Source: CAD feature listing. Evaluate the final solid. Frame: model axes, mm. A direction names the side the tool comes from. Round coordinates to 2 decimals unless told otherwise and drop trailing zeros. Loops run counter-clockwise (first coordinate to the right, second up) from the corner with the lowest first, then second, coordinate; pieces in that order, holes last. Notation, with made-up numbers: M -30.75,44 L -6.75,44 A8 ccw -6.75,58 Z; hole C 65,36.5 d3. An arc over 180 degrees is marked long. One line per item, written item: value.
from build123d import *

# Parameters (mm, degrees)
SKETCH1_R                  = 109.714317711
SKETCH1_R_2                = 85.130943159
BOSS_EXTRUDE1_DEPTH        = 50
BOSS_EXTRUDE2_REACH        = 241.217
BOSS_EXTRUDE2_START_RADIUS = 109.714317711
BOSS_EXTRUDE2_END_RADIUS   = 109.714317711
SKETCH2_W                  = 26
SKETCH2_H                  = 26
SKETCH2_W_2                = 20
SKETCH2_H_2                = 20


with BuildPart() as part:
    # Sketch1 → Boss-Extrude1 (new body)
    with BuildSketch(Plane.XY):
        Circle(SKETCH1_R)
        Circle(SKETCH1_R_2, mode=Mode.SUBTRACT)
    extrude(amount=BOSS_EXTRUDE1_DEPTH)

    # Boss-Extrude2: from a cylinder face, 241.217 long prism both ways, kept between that surface and its translate by the depth
    boss_extrude2_start = Plane(origin=(0, 0, 25), z_dir=(0, 0, -1)) * Cylinder(BOSS_EXTRUDE2_START_RADIUS, 702.862635421, mode=Mode.PRIVATE)
    boss_extrude2_end = Plane(origin=(76.2, 0, 25), z_dir=(0, 0, -1)) * Cylinder(BOSS_EXTRUDE2_END_RADIUS, 702.862635421, mode=Mode.PRIVATE)
    # Sketch2 → Boss-Extrude2 (add, from a surface)
    with BuildSketch(Plane(origin=(0, 0, 0), x_dir=(0, 0, -1), z_dir=(1, 0, 0)), mode=Mode.PRIVATE) as boss_extrude2_sk1:
        with Locations((-25, 0)):
            Rectangle(SKETCH2_W, SKETCH2_H)
        with Locations((-25, 0)):
            Rectangle(SKETCH2_W_2, SKETCH2_H_2, mode=Mode.SUBTRACT)
    boss_extrude2_tool1 = extrude(boss_extrude2_sk1.sketch, amount=BOSS_EXTRUDE2_REACH, both=True, mode=Mode.PRIVATE)
    add(((boss_extrude2_tool1 - boss_extrude2_start) & boss_extrude2_end).solids().sort_by_distance((147.199526, 12.632304, 25))[0])


solid = part.part
1. Section query D-D (x = 0). Return the cut outline in (y, z), and give its area (3 significant figures).
Report:
outline: M -109.71,0 L -85.13,0 L -85.13,50 L -109.71,50 Z; M 85.13,0 L 109.71,0 L 109.71,50 L 85.13,50 Z
area: 2,460 mm2
2. Section query A-A (z = 29). Return the cut outline in (x, y).
Report:
outline: M 108.94,-13 L 185.14,-13 A109.71 ccw 185.46,-10 L 109.26,-10 A109.71 ccw 109.26,10 L 185.46,10 A109.71 ccw 185.14,13 L 108.94,13 A109.71 ccw long Z; hole C 0,0 d170.26
3. Ray query, line 1 (Z direction, x = 173, y = 2); line 2 (Y direction, x = 0, z = 33); line 3 (Y direction, x = 139.5, z = 21.5). Return the intervals inside material, ascending. Write a range as [from, to].
Report:
line 1: z = [12, 15], [35, 38]
line 2: y = [-109.71, -85.13], [85.13, 109.71]
line 3: y = [-13, -10], [10, 13]
4. Section query B-B (x = 163). Return the cut outline in (y, z).
Report:
outline: M -13,12 L 13,12 L 13,38 L -13,38 Z; hole M -10,15 L 10,15 L 10,35 L -10,35 Z
5. Reachability of faces 1 (the face through (148, 0, 15)), 2 (the face through (148, 0, 12)), 3 (the face through (148, 13, 25)) from +Z, -Z, +X, -X, +Y, -Y: full face, straight path, thin tool, end or side. Return the list, or none.
Report:
face 1: +X
face 2: -Z, +X, +Y, -Y
face 3: +Z, -Z, +X, +Y
6. Section query C-C (y = 0). Return the cut outline in (x, z), and give its area (3 significant figures).
Report:
outline: M -109.71,0 L -85.13,0 L -85.13,50 L -109.71,50 Z; M 85.13,0 L 109.71,0 L 109.71,12 L 185.91,12 L 185.91,15 L 109.71,15 L 109.71,35 L 185.91,35 L 185.91,38 L 109.71,38 L 109.71,50 L 85.13,50 Z
area: 2,920 mm2
7. Pin query (flat end, axial travel): pin 1 (1 mm diameter, centred on y = 26, z = 13.5, fed in from -X); pin 2 (10 mm diameter, centred on x = 128.5, z = 27, fed in from -Y); pin 3 (22 mm diameter, centred on x = 152.5, z = 23.5, fed in from +Y). Return the tip coordinate at first contact, or that it passes through.
Report:
pin 1: stops at x = -106.71
pin 2: stops at y = -13
pin 3: stops at y = 13
8. Pull-direction query (Y, two-part tool) for faces 4 (the face through (148, 0, 38)), 5 (the face through (148, -10, 25)), 6 (the face through (148, -13, 25)); classes: released by +Y, released by -Y, zero draft, split by the parting line, or undercut.
Report:
face 4: zero draft
face 5: undercut
face 6: released by -Y
